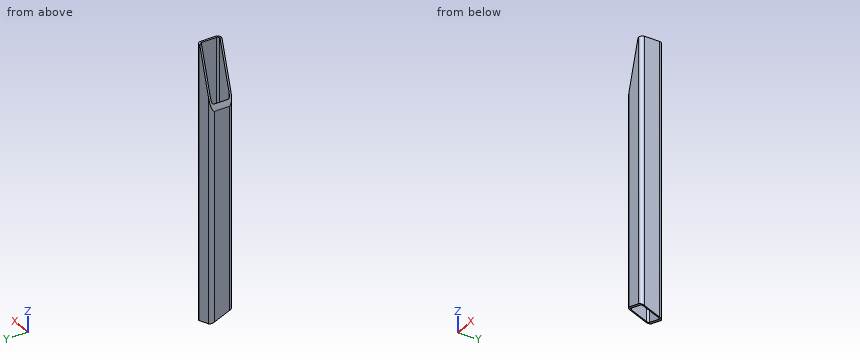
```python
from build123d import *

# Parameters (mm, degrees)
BOSS_EXTRUDE1_DEPTH     = 584.2
CUT_EXTRUDE1_DEPTH      = 1168.4
CUT_EXTRUDE1_DEPTH_BACK = 587.679520693
CUT_EXTRUDE2_DEPTH      = 587.679520693
CUT_EXTRUDE2_DEPTH_BACK = 587.679520693
CUT_EXTRUDE3_DEPTH      = 591.379276398


with BuildPart() as part:
    # Sketch1 → Boss-Extrude1 (new, symmetric)
    with BuildSketch(Plane.XY):
        with BuildLine():
            Line((-25.4, -38.1), (25.4, -38.1))
            ThreePointArc((25.4, -38.1), (34.380256121, -34.380256121), (38.1, -25.4))
            Line((38.1, -25.4), (38.1, 25.4))
            ThreePointArc((38.1, 25.4), (34.380256121, 34.380256121), (25.4, 38.1))
            Line((25.4, 38.1), (-25.4, 38.1))
            ThreePointArc((-25.4, 38.1), (-34.380256121, 34.380256121), (-38.1, 25.4))
            Line((-38.1, 25.4), (-38.1, -25.4))
            ThreePointArc((-38.1, -25.4), (-34.380256121, -34.380256121), (-25.4, -38.1))
        make_face()
        with BuildLine():
            Line((-25.4, 31.75), (25.4, 31.75))
            ThreePointArc((25.4, 31.75), (29.890128061, 29.890128061), (31.75, 25.4))
            Line((31.75, 25.4), (31.75, -25.4))
            ThreePointArc((31.75, -25.4), (29.890128061, -29.890128061), (25.4, -31.75))
            Line((25.4, -31.75), (-25.4, -31.75))
            ThreePointArc((-25.4, -31.75), (-29.890128061, -29.890128061), (-31.75, -25.4))
            Line((-31.75, -25.4), (-31.75, 25.4))
            ThreePointArc((-31.75, 25.4), (-29.890128061, 29.890128061), (-25.4, 31.75))
        make_face(mode=Mode.SUBTRACT)
    extrude(amount=BOSS_EXTRUDE1_DEPTH, both=True)

    # Sketch2 → Cut-Extrude1 (cut, two sides: drawn at the far end of the back side and taken through both)
    with BuildSketch(Plane(origin=(0, 0, 0), x_dir=(1, 0, 0), z_dir=(0, 1, 0)).offset(-CUT_EXTRUDE1_DEPTH_BACK)):
        Polygon((-38.1, -584.2), (38.1, -584.2), (-38.1, -334.961030472), align=None)
    extrude(amount=CUT_EXTRUDE1_DEPTH + CUT_EXTRUDE1_DEPTH_BACK, mode=Mode.SUBTRACT)

    # Sketch3 → Cut-Extrude2 (cut, two sides: drawn at the far end of the back side and taken through both)
    with BuildSketch(Plane(origin=(0, 0, 0), x_dir=(0, 0, -1), z_dir=(1, 0, 0)).offset(-CUT_EXTRUDE2_DEPTH_BACK)):
        Polygon((529.224802616, 234.912944521), (393.7, -38.1), (621.210787101, -151.037335513), (756.735589716, 121.975609008), align=None)
    extrude(amount=CUT_EXTRUDE2_DEPTH + CUT_EXTRUDE2_DEPTH_BACK, mode=Mode.SUBTRACT)

    # Sketch4 → Cut-Extrude3 (cut, through all)
    with BuildSketch(Plane(origin=(0, 38.1, 0), x_dir=(1, 0, 0), z_dir=(0, 1, 0))):
        Polygon((22.568881382, -533.4), (38.1, -533.4), (38.1, -584.2), align=None)
    extrude(amount=-CUT_EXTRUDE3_DEPTH, mode=Mode.SUBTRACT)

    # SurfaceCut1
    split(bisect_by=Plane(origin=(-91.776590451, -128.480237958, -300.187701194), x_dir=(0.9626963442251767, -0.1064681232735412, -0.24875748740910325), z_dir=(0.2705840882525802, 0.37879711890625634, 0.885040673581073)), keep=Keep.TOP)


solid = part.part
```
Verification items for the finished model (mm, model axes). Coordinates: 2 decimals unless noted, no trailing zeros. Write each loop counter-clockwise with the first axis right and the second up, starting at its lowest first coordinate (ties: lowest second). Pieces come first, ordered by that corner, then holes. Notation, with made-up numbers: (-30.5, 17) - (-19.5, 17) arc R9 ccw to (-19.5, 34) - close; hole circle Ø10 at (86, -3.5). An arc over 180 degrees is marked (long way). Write item = value, one per line.
Q1. Cross-section at A-A (x = 14). Enter the section's corners in (y, z), plus the area to 3 significant figures.
Answer:
outline = (-38.1, -371.21) - (-31.75, -373.93) - (-31.75, 505.37) - (-38.1, 505.37) - close; (31.75, -401.11) - (38.1, -403.82) - (38.1, 505.37) - (31.75, 505.37) - close
area = 11,300 mm²
Q2. Cross-section at B-B (y = -16.5). Enter the section's corners in (x, z), plus the area to 3 significant figures.
Answer:
outline = (-38.1, -364.53) - (-31.75, -366.47) - (-31.75, 355.73) - (-38.1, 334.96) - close; (31.75, -385.88) - (38.1, -387.82) - (38.1, 533.4) - (31.75, 533.4) - close
area = 10,400 mm²
Q3. Cross-section at C-C (z = -188.5). Enter the section's corners in (x, y), plus the area to 3 significant figures.
Answer:
outline = (-38.1, -25.4) arc R12.7 ccw to (-25.4, -38.1) - (25.4, -38.1) arc R12.7 ccw to (38.1, -25.4) - (38.1, 25.4) arc R12.7 ccw to (25.4, 38.1) - (-25.4, 38.1) arc R12.7 ccw to (-38.1, 25.4) - close; hole (-31.75, -25.4) arc R6.35 ccw to (-25.4, -31.75) - (25.4, -31.75) arc R6.35 ccw to (31.75, -25.4) - (31.75, 25.4) arc R6.35 ccw to (25.4, 31.75) - (-25.4, 31.75) arc R6.35 ccw to (-31.75, 25.4) - close
area = 1,670 mm²
Q4. Material ranges on L1, parallel to X at y = -20.5, z = 226; L2, parallel to Y at x = 27.5, z = 441.5, recorded low to high. Write a range as from..to.
Answer:
L1 = -38.1..-31.75, 31.75..38.1
L2 = -37.93..-31.39, 31.39..37.93
Q5. Cross-section at D-D (z = 348). Enter the section's corners in (x, y), plus the area to 3 significant figures.
Answer:
outline = (-34.11, -34.64) arc R12.7 ccw to (-25.4, -38.1) - (25.4, -38.1) arc R12.7 ccw to (38.1, -25.4) - (38.1, 25.4) arc R12.7 ccw to (25.4, 38.1) - (-25.4, 38.1) arc R12.7 ccw to (-34.11, 34.64) - close; hole (-31.75, -25.4) arc R6.35 ccw to (-25.4, -31.75) - (25.4, -31.75) arc R6.35 ccw to (31.75, -25.4) - (31.75, 25.4) arc R6.35 ccw to (25.4, 31.75) - (-25.4, 31.75) arc R6.35 ccw to (-31.75, 25.4) - close
area = 1,420 mm²
Q6. Go/stop test with a flat-tipped pin: pin 1 Ø10 at (x, y) = (-25.5, 18) entering from -Z. Record where the tip stops, or that it passes through.
Answer:
pin_1 = through
